Autodesk Inventor part; units mm, degrees
ref_plane "YZ Plane" through (0, 0, 0) normal (1, 0, 0) x (0, 1, 0)
ref_plane "XZ Plane" through (0, 0, 0) normal (0, 1, 0) x (-1, 0, 0)
ref_plane "XY Plane" through (0, 0, 0) normal (0, 0, 1) x (1, 0, 0)
sketch "Sketch1" plane through (0, 0, 0) normal (0, 0, 1) x (1, 0, 0)
  circle A0 centre (0, 0) radius 3.175
  circle A1 centre (0, 0) radius 6.35
  line L0 (-5.967, 2.1718) -> (-76.0939, -190.5)
  line L1 (-76.0939, -190.5) -> (76.0939, -190.5)
  line L2 (76.0939, -190.5) -> (5.967, 2.1718)
  line L3 (0, -18.5662) -> (-57.9564, -177.8)
  line L4 (-57.9564, -177.8) -> (57.9564, -177.8)
  line L5 (57.9564, -177.8) -> (0, -18.5662)
  dimension "d0" = 6.35
  dimension "d1" = 12.7
  dimension "d2" = 70
  dimension "d3" = 70
  dimension "d4" = 190.5
  dimension "d5" = 12.7
  dimension "d9" = 152.1877
extrude "Extrusion1" add sketch "Sketch1" along normal blind 6.35
fillet "Fillet1" radius 3.175 3 edges at (0, -18.5662, 3.175) (-57.9564, -177.8, 3.175) (57.9564, -177.8, 3.175)
sketch "Sketch2" plane through (-76.0939, -190.5, 0) normal (0, -1, 0) x (1, 0, 0)
  circle A0 centre (19.05, 3.175) radius 1.5875
  circle A1 centre (133.1377, 3.175) radius 1.5875
  line L0 (0, 6.35) -> (152.1877, 6.35)
  line L1 (0, 0) -> (0, 6.35)
  line L2 (152.1877, 0) -> (152.1877, 6.35)
  point P0 (76.0939, 0)
  dimension "d10" = 3.175
  dimension "d11" = 3.175
  dimension "d12" = 19.05
  dimension "d13" = 19.05
extrude "Extrusion2" add sketch "Sketch2" along normal blind 6.35
properties part number "Outside"
Build history of the part. All positions in model axes, mm. A direction names the side the tool comes from. Round coordinates to 2 decimals unless told otherwise and drop trailing zeros. Order: outer loops, then holes, each group sorted by start corner. A loop starts at its lowest first (then second) coordinate and runs counter-clockwise, first axis right, second up. Notation, with made-up numbers: M -2,79 L 56,79 A14 ccw 56,93 Z; hole C -36,21 d7. An arc over 180 degrees is marked long. Use CSV: the item, a comma, the result in double quotes. Start each with the question number.
(1) Cut at A-A on x = 0. List the corners of the cut face in (y, z) (3 decimals), then the cut area to 3 significant figures.
(2) Cut at B-B on x = -25.5. List the corners of the cut face in (y, z), then the cut area to 3 significant figures.
(3) Tool access for faces 1 (the face through (-0.11, 6.35, 3.13)), 2 (the face through (56, -176.48, 3.22)): list every direction of +Z, -Z, +X, -X, +Y, -Y with a clear straight run to the whole face (end or side of a thin tool).
(4) Mould opens along X. For faces 3 (the face through (41.52, -95.51, 3.13)), 4 (the face through (-0.69, 3.1, 3.13)), 5 (the face through (-40.54, -92.82, 3.13)) say: +X half, -X half, draft (parallel to the pull), parting line (faces both ways), or undercut.
(5) Flat gauge pins, fed straight in: P1, Ø1, axis at y = -96.5, z = 2, coming from the +X side; P2, Ø1.5, axis at y = -168, z = 5, coming from the +X side; P3, Ø3, axis at x = 30.5, z = 3, coming from the -Y side. Where does each tip first touch, or does it go through?
(6) Cut at C-C on y = -164. List the corners of the cut face in (x, z).
(7) Drill centre lines: probe 1 along X at (y, z) = (-47, 4); probe 2 along X at (y, z) = (-61, 5.25); probe 3 along X at (y, z) = (-188, 3.75). Where is each one in solid material? Low to high.
Findings:
1,outline,"M -190.5,0 L -177.8,0 L -177.8,6.35 L -190.5,6.35 Z; M -24.674,0 L -3.175,0 L -3.175,6.35 L -24.674,6.35 Z; M 3.175,0 L 6.35,0 L 6.35,6.35 L 3.175,6.35 Z"
1,area,"237 mm^2"
2,outline,"M -190.5,0 L -177.8,0 L -177.8,6.35 L -190.5,6.35 Z; M -88.63,0 L -51.49,0 L -51.49,6.35 L -88.63,6.35 Z"
2,area,"316 mm^2"
3,face 1,"+Z, -Z, +Y"
3,face 2,"+Z, -Z"
4,face 3,"+X half"
4,face 4,"undercut"
4,face 5,"-X half"
5,P1,"stops at x = 42.06"
5,P2,"stops at x = 68.18"
5,P3,"stops at y = -190.5"
6,outline,"M -66.45,0 L -52.93,0 L -52.93,6.35 L -66.45,6.35 Z; M 52.93,0 L 66.45,0 L 66.45,6.35 L 52.93,6.35 Z"
7,probe 1,"x = -23.86 to -10.35, 10.35 to 23.86"
7,probe 2,"x = -28.96 to -15.44, 15.44 to 28.96"
7,probe 3,"x = -75.18 to 75.18"
